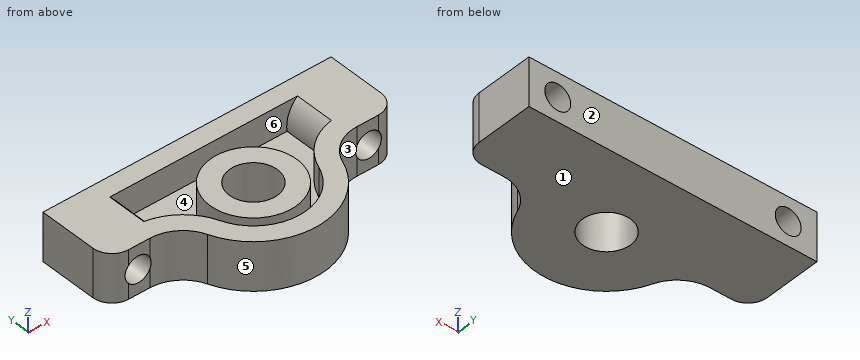
from build123d import *

# Parameters (mm, degrees)
F1_DEPTH    = 6.35
F2_R        = 5.08
F3_R        = 1.7145
F5_DEPTH    = 19.686
F6_T        = 2.54
F7_T1_DEPTH = 19.05


# Not quite as in the source:
# - a fillet or chamfer that OpenCascade refuses, or shapes differently, is made with other operations: its cross-section is extruded or revolved along the edge and cut away or added
# - a shell that OpenCascade refuses in one call is made with other operations: the cavity is built on its own and cut out
# - a feature names something its author has since deleted; it is built from what else it names


with BuildPart() as f1:
    # F0 (on Top) → F1 (new body)
    with BuildSketch(Plane.XY):
        with BuildLine():
            Line((9.525, 0), (3.175, 0))
            ThreePointArc((3.175, 0), (0, -3.175), (-3.175, 0))
            Line((-3.175, 0), (-9.525, 0))
            ThreePointArc((-9.525, 0), (0, -9.525), (9.525, 0))
        make_face()
        with BuildLine():
            ThreePointArc((-3.175, 0), (0, 3.175), (3.175, 0))
            Line((3.175, 0), (9.525, 0))
            ThreePointArc((9.525, 0), (0, 9.525), (-9.525, 0))
            Line((-9.525, 0), (-3.175, 0))
        make_face()
        with BuildLine():
            ThreePointArc((-9.525, 0), (0, 9.525), (9.525, 0))
            Line((9.525, 0), (19.05, 0))
            Line((19.05, 0), (19.05, 10.16))
            Line((19.05, 10.16), (-19.05, 10.16))
            Line((-19.05, 10.16), (-19.05, 0))
            Line((-19.05, 0), (-9.525, 0))
        make_face()
    extrude(amount=F1_DEPTH)

    # F2
    f2_edges = [f1.edges().sort_by_distance(p)[0] for p in [
        (9.525, 0, 3.175),
        (-9.525, 0, 3.175),
    ]]
    fillet(f2_edges, radius=F2_R)

    # F3 (on face) → F5 (cut, through all)
    with BuildSketch(Plane(origin=(0, 10.16, 0), x_dir=(-1, 0, 0), z_dir=(0, 1, 0))):
        with Locations((15.24, 3.175)):
            Circle(F3_R)
        with Locations((-15.24, 3.175)):
            Circle(F3_R)
    extrude(amount=-F5_DEPTH, mode=Mode.SUBTRACT)

    # F6: shell of thickness 2.54, made by hand


with BuildPart() as f6_core1:
    # F6_t2: copy of F1
    add(f1.part)

    # the walls: a layer under each face that stays
    f6_faces = [f6_core1.faces().sort_by_distance(p)[0] for p in [
        (0, -9.525, 3.175),
        (-12.7, 0.3175, 0),
        (-10.7921658217, -0.9097158891, 3.175),
        (10.7921658217, -0.9097158891, 3.175),
        (-18.1571750408, 0, 5.2916666667),
        (14.5858752038, 0, 5.2916666667),
        (-19.05, 5.08, 3.175),
        (19.05, 5.08, 3.175),
        (0, 10.16, 3.175),
        (3.175, 0, 3.175),
        (-13.5255, 5.0786180746, 3.175),
        (16.9545, 5.0786180746, 3.175),
    ]]
    thicken(f6_faces, amount=-F6_T, mode=Mode.SUBTRACT)


with BuildPart() as f1_1:
    add(f1.part)

    # what is left inside the walls is the cavity
    f6_cavity = [f6_core1.part.solids().sort_by_distance(p)[0] for p in [
        (-6.204007, 2.751667, 6.3246),
    ]]
    add(f6_cavity, mode=Mode.SUBTRACT)

    # F7: fillet of radius 2.54 on 2 edges, made by hand

    # F7_s2 → F7_t1 (cut)
    with BuildSketch(Plane.XY.offset(-6.35)):
        with BuildLine():
            ThreePointArc((-16.51, 0), (-18.3060512242, 0.7439487758), (-19.05, 2.54))
            Line((-19.05, 2.54), (-19.05, 0))
            Line((-19.05, 0), (-16.51, 0))
        make_face()
        with BuildLine():
            ThreePointArc((16.51, 0), (18.3060512242, 0.7439487758), (19.05, 2.54))
            Line((19.05, 2.54), (19.05, 0))
            Line((19.05, 0), (16.51, 0))
        make_face()
    extrude(amount=F7_T1_DEPTH, mode=Mode.SUBTRACT)


solid = f1_1.part
Read the model definition and answer for the solid it produces. Units are mm, in the model's axes. Face numbers are marked on the shaded views. A direction names the side the tool comes from. Round coordinates to 2 decimals unless told otherwise and drop trailing zeros. Loops run counter-clockwise (first coordinate to the right, second up) from the corner with the lowest first, then second, coordinate; pieces in that order, holes last.
Q1. Which of the six approach directions +Z, -Z, +X, -X, +Y, -Y give full straight-line access (tool end or side, diameter ignored) to the marked faces 5 and 6?
Q2. Section A-A on x = 0 is taken. Write down the section's boundary in (y, z) (3 decimals).
Q3. Section B-B on z = 0.5 is taken. Write down the section's boundary in (x, y) (3 decimals).
Q4. Consider probe 1 along Y at (x, z) = (0, 4.25) (3 decimals); probe 2 along Y at (x, z) = (0, 2) (3 decimals); probe 3 along Y at (x, z) = (-2, 5). Determine where each line is inside the solid, lowest interval first.
Q5. Section C-C on y = -1.25 is taken. Write down the section's boundary in (x, z), and give its area (3 significant figures).
Q6. Each of these flat-tipped pins is pushed along its axis until it touches: pin 1 (5 mm diameter, centred on x = 0, y = 0, fed in from +Z); pin 2 (1.9 mm diameter, centred on x = 15, z = 5, fed in from -Y); pin 3 (1.5 mm diameter, centred on x = -1.5, z = 1, fed in from -Y); pin 4 (2 mm diameter, centred on y = -3.5, z = 1.5, fed in from +X). Where does it stop, or does it pass through?
Q7. Determine the mould class of the marked faces 1, 2, 3 and 4 for opening direction Y: released by +Y, released by -Y, zero draft, split by the parting line, or undercut.
Q8. Section D-D on z = 5.25 is taken. Write down the section's boundary in (x, y) (3 decimals), and give its area (3 significant figures).
Output:
1. face 5: +Z, -Z, -Y
1. face 6: +Z
2. outline: (-9.525, 0) - (-3.175, 0) - (-3.175, 6.35) - (-5.715, 6.35) - (-5.715, 2.54) - (-6.985, 2.54) - (-6.985, 6.35) - (-9.525, 6.35) - close; (3.175, 0) - (10.16, 0) - (10.16, 6.35) - (7.62, 6.35) - (7.62, 2.54) - (5.715, 2.54) - (5.715, 6.35) - (3.175, 6.35) - close
3. outline: (-19.05, 2.54) arc R2.54 ccw to (-16.51, 0) - (-13.693, 0) arc R5.08 cw to (-8.93, -3.313) arc R9.525 ccw to (8.93, -3.313) arc R5.08 cw to (13.693, 0) - (16.51, 0) arc R2.54 ccw to (19.05, 2.54) - (19.05, 10.16) - (-19.05, 10.16) - close; hole circle Ø6.35 at (0, 0)
4. probe 1: y = -9.525 to -6.985, -5.715 to -3.175, 3.175 to 5.715, 7.62 to 10.16
4. probe 2: y = -9.525 to -3.175, 3.175 to 10.16
4. probe 3: y = -9.31 to -6.69, -5.35 to -2.47, 2.47 to 5.35, 7.62 to 10.16
5. outline: (-10.36, 0) - (-2.92, 0) - (-2.92, 6.35) - (-5.58, 6.35) - (-5.58, 2.54) - (-7.11, 2.54) - (-7.11, 6.35) - (-10.36, 6.35) - close; (2.92, 0) - (10.36, 0) - (10.36, 6.35) - (7.11, 6.35) - (7.11, 2.54) - (5.58, 2.54) - (5.58, 6.35) - (2.92, 6.35) - close
5. area: 82.8 mm2
6. pin 1: passes through
6. pin 2: stops at y = 0
6. pin 3: stops at y = -9.5
6. pin 4: stops at x = 9.32
7. face 1: zero draft
7. face 2: released by +Y
7. face 3: released by -Y
7. face 4: undercut
8. outline: (-19.05, 2.54) arc R2.54 ccw to (-16.51, 0) - (-13.693, 0) arc R5.08 cw to (-8.93, -3.313) arc R9.525 ccw to (8.93, -3.313) arc R5.08 cw to (13.693, 0) - (16.51, 0) arc R2.54 ccw to (19.05, 2.54) - (19.05, 10.16) - (-19.05, 10.16) - close; circle Ø11.43 at (0, 0); hole (-11.526, 2.225) arc R7.62 cw to (-6.549, -2.43) arc R6.985 ccw to (6.549, -2.43) arc R7.62 cw to (11.526, 2.225) - (11.526, 7.62) - (-11.526, 7.62) - close; hole circle Ø6.35 at (0, 0)
8. area: 359 mm2
